Check sheet for the modelled part. Datum: model origin and axes. Units: mm. Face numbers are marked on the shaded views. A direction names the side the tool comes from. Give positions to 0.01 mm unless a question says otherwise; leave off trailing zeros. Write each loop counter-clockwise with the first axis right and the second up, starting at its lowest first coordinate (ties: lowest second). Pieces come first, ordered by that corner, then holes. Notation, with made-up numbers: (-38, 8) -> (-6, 8) arc R32 ccw to (-6, 45) -> close; hole circle Ø2 at (49.25, -15.75). An arc over 180 degrees is marked (long way). Return JSON: item names as keys, results as strings.
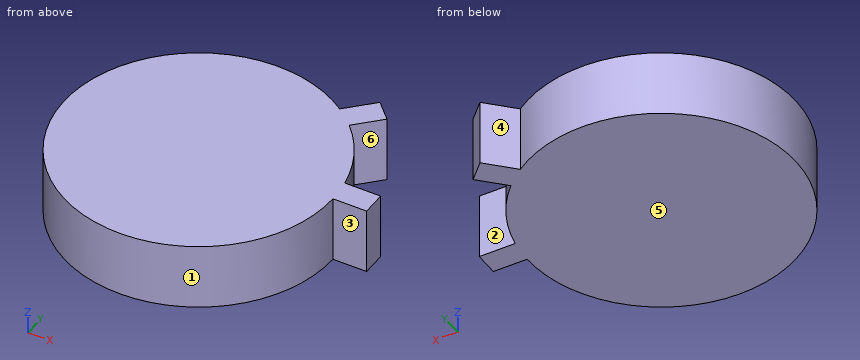
from build123d import *

# Parameters (mm, degrees)
F1_DEPTH = 25


with BuildPart() as f1:
    # F0 (on Top) → F1 (new body)
    with BuildSketch(Plane.XY):
        with BuildLine():
            Line((0, 0), (50.35, 0))
            ThreePointArc((50.35, 0), (50.146865, 4.518229), (49.539101, 9))
            ThreePointArc((49.539101, 9), (44.600611, 23.364673), (35.602826, 35.602826))
            Line((35.602826, 35.602826), (0, 0))
        make_face()
        with BuildLine():
            ThreePointArc((28.665473, 41.393395), (-44.600611, -23.364673), (50.35, 0))
            Line((50.35, 0), (0, 0))
            Line((0, 0), (35.602826, 35.602826))
            ThreePointArc((35.602826, 35.602826), (32.264319, 38.654059), (28.665473, 41.393395))
        make_face()
        with BuildLine():
            ThreePointArc((49.539101, 9), (50.146865, 4.518229), (50.35, 0))
            Line((50.35, 0), (63, 0))
            Line((63, 0), (63, 9))
            Line((63, 9), (49.539101, 9))
        make_face()
        with BuildLine():
            Line((38.183766, 50.911688), (28.665473, 41.393395))
            ThreePointArc((28.665473, 41.393395), (32.264319, 38.654059), (35.602826, 35.602826))
            Line((35.602826, 35.602826), (44.547727, 44.547727))
            Line((44.547727, 44.547727), (38.183766, 50.911688))
        make_face()
    extrude(amount=F1_DEPTH)


solid = f1.part
(1) Cross-section at D-D on x = 15. Enter the section's corners in (y, z).
Reply:
{"outline": "(-48.06, 0) -> (48.06, 0) -> (48.06, 25) -> (-48.06, 25) -> close"}
(2) Thickness scan on L1, parallel to Y at x = 56.5, z = 10.5; L2, parallel to X at y = 1.5, z = 18.75; L3, parallel to Y at x = 2.5, z = 4. Record the ranges inside material, lowest first.
Reply:
{"L1": "0 to 9", "L2": "-50.33 to 63", "L3": "-50.29 to 50.29"}
(3) Cross-section at A-A on z = 15. Enter the section's corners in (x, y).
Reply:
{"outline": "(28.67, 41.39) arc R50.35 ccw (long way) to (50.35, 0) -> (63, 0) -> (63, 9) -> (49.54, 9) arc R50.35 ccw to (35.6, 35.6) -> (44.55, 44.55) -> (38.18, 50.91) -> close"}
(4) Release check for a two-part mould opening along Y. For the marked faces 3, 4, 5 and 6 record: pulls with the +Y half, pulls with the -Y half, needs draft (parallel to the pull), parting line crosses it, or undercut.
Reply:
{"face 3": "pulls with the -Y half", "face 4": "pulls with the +Y half", "face 5": "needs draft", "face 6": "undercut"}
(5) Cross-section at C-C on y = -8. Enter the section's corners in (x, z), then the cut area to 3 significant figures.
Reply:
{"outline": "(-49.71, 0) -> (49.71, 0) -> (49.71, 25) -> (-49.71, 25) -> close", "area": "2,490 mm^2"}
(6) Set-up check for the marked faces 1 and 2: record each of +Z, -Z, +X, -X, +Y, -Y from which the full face is reachable in a straight line by a thin tool's end or side.
Reply:
{"face 1": "+Z, -Z", "face 2": "+Z, -Z, +X, +Y"}
(7) Cross-section at B-B on x = 40.5. Enter the section's corners in (y, z).
Reply:
{"outline": "(-29.91, 0) -> (29.91, 0) -> (29.91, 25) -> (-29.91, 25) -> close; (40.5, 0) -> (48.6, 0) -> (48.6, 25) -> (40.5, 25) -> close"}
(8) Depth check by flat-ended pin: pin 1 Ø10 at (y, z) = (22.5, 8.5) entering from +X; pin 2 Ø11 at (x, z) = (58, 10) entering from +Y; pin 3 Ø4 at (x, z) = (-9.5, 16) entering from -Y. Enter the tip coordinate at first touch or a pass-through.
Reply:
{"pin 1": "x = 47.21", "pin 2": "y = 9", "pin 3": "y = -49.79"}
